from build123d import *

# Parameters (mm, degrees)
SKETCH_1_R          = 15
EXTRUDE_1_DEPTH     = 5.65
SKETCH_2_R          = 10
EXTRUDE_2_DEPTH     = 46.4
SKETCH_3_R          = 1.25
CUT_EXTRUDE_1_DEPTH = 10
SKETCH_4_OUTSIDE_W  = 45.43
SKETCH_4_OUTSIDE_H  = 45.43
SKETCH_4_OUTSIDE_R  = 7.5
CUT_EXTRUDE_2_DEPTH = 7
SKETCH_5_OUTSIDE_W  = 45.43
SKETCH_5_OUTSIDE_H  = 45.43
SKETCH_5_OUTSIDE_R  = 8.5
CUT_EXTRUDE_3_DEPTH = 1
SKETCH_6_R          = 1.4
CUT_EXTRUDE_4_DEPTH = 8
CUT_EXTRUDE_5_DEPTH = 3


with BuildPart() as part:
    # 草图1 → 凸台-拉伸1 (new body)
    with BuildSketch(Plane.XY):
        Circle(SKETCH_1_R)
    extrude(amount=EXTRUDE_1_DEPTH)

    # 草图2 → 凸台-拉伸2 (add)
    with BuildSketch(Plane.XY.offset(5.65)):
        Circle(SKETCH_2_R)
    extrude(amount=EXTRUDE_2_DEPTH)

    # 草图3 → 切除-拉伸1 (cut)
    with BuildSketch(Plane(origin=(0, 0, 0), x_dir=(-1, 0, 0), z_dir=(0, 0, -1))):
        with Locations((0, 7)):
            Circle(SKETCH_3_R)
        with Locations((7, 0)):
            Circle(SKETCH_3_R)
        with Locations((0, -7)):
            Circle(SKETCH_3_R)
        with Locations((-7, 0)):
            Circle(SKETCH_3_R)
    extrude(amount=-CUT_EXTRUDE_1_DEPTH, mode=Mode.SUBTRACT)

    # 草图4 outside → 切除-拉伸2 (cut)
    with BuildSketch(Plane.XY.offset(52.05)):
        Rectangle(SKETCH_4_OUTSIDE_W, SKETCH_4_OUTSIDE_H)
        Circle(SKETCH_4_OUTSIDE_R, mode=Mode.SUBTRACT)
    extrude(amount=-CUT_EXTRUDE_2_DEPTH, mode=Mode.SUBTRACT)

    # 草图5 outside → 切除-拉伸3 (cut)
    with BuildSketch(Plane.XY.offset(45.05)):
        Rectangle(SKETCH_5_OUTSIDE_W, SKETCH_5_OUTSIDE_H)
        Circle(SKETCH_5_OUTSIDE_R, mode=Mode.SUBTRACT)
    extrude(amount=-CUT_EXTRUDE_3_DEPTH, mode=Mode.SUBTRACT)

    # 草图6 → 切除-拉伸4 (cut)
    with BuildSketch(Plane(origin=(0, 10, 0), x_dir=(1, 0, 0), z_dir=(0, 1, 0))):
        with Locations(Location((0, -39.65, 0), (0, 0, 270))):
            Circle(SKETCH_6_R)
    cut_extrude_4 = extrude(amount=-CUT_EXTRUDE_4_DEPTH, mode=Mode.SUBTRACT)

    # 镜向1: 切除-拉伸4 across plane
    add(cut_extrude_4.mirror(Plane.ZX), mode=Mode.SUBTRACT)

    # 草图7 → 切除-拉伸5 (cut)
    with BuildSketch(Plane(origin=(10, 0, 0), x_dir=(0, 0, -1), z_dir=(1, 0, 0))):
        with BuildLine():
            Line((-32.15, 2.6), (-15.65, 2.6))
            ThreePointArc((-15.65, 2.6), (-13.05, 0), (-15.65, -2.6))
            Line((-15.65, -2.6), (-32.15, -2.6))
            ThreePointArc((-32.15, -2.6), (-34.75, 0), (-32.15, 2.6))
        make_face()
    extrude(amount=-CUT_EXTRUDE_5_DEPTH, mode=Mode.SUBTRACT)


solid = part.part
Could you check a few things on this model? Use its own coordinates, in mm. A direction names the side the tool comes from. Round coordinates to 2 decimals unless told otherwise and drop trailing zeros. Order: outer loops, then holes, each group sorted by start corner. A loop starts at its lowest first (then second) coordinate and runs counter-clockwise, first axis right, second up.
(1) Please list where these lines run through material, in increasing order: line 1 along Z through (x, y) = (0, -7.75); line 2 along X through (y, z) = (-5.25, 39.65); line 3 along Z through (x, y) = (12, -0.5).
Response values:
line 1: z = 10 to 38.25, 41.05 to 45.05
line 2: x = -8.51 to -1.4, 1.4 to 8.51
line 3: z = 0 to 5.65
(2) Imagine slicing it at D-D (z = 25.5). Write out the boundary of the cut face in (x, y), plus the area to 3 significant figures.
Response values:
outline: (7, -2.6) - (7, 2.6) - (9.66, 2.6) arc R10 ccw (long way) to (9.66, -2.6) - close
area: 299 mm2
(3) Imagine slicing it at B-B (z = 36.5). Write out the boundary of the cut face in (x, y).
Response values:
outline: circle Ø20 at (0, 0)
(4) Which directions (+Z, -Z, +X, -X, +Y, -Y) give clear straight access to the entire face, cutting with the end or side of a thin tool? Please do faces 1 (the cylindrical face through (-14.985, 0.66, 2.785)), 2 (the cylindrical face through (0.27, 5.78, 4.93)), 3 (the flat face through (0, 0, 0)), 4 (the cylindrical face through (8.52, -0.06, 34.75)), 5 (the cylindrical face through (-2.17, -9.76, 24.58)).
Response values:
face 1: +Z, -Z
face 2: -Z
face 3: -Z, +X, -X, +Y, -Y
face 4: +X
face 5: +Z
(5) I'm going to push flat-ended pins straight in: pin 1 (2 mm diameter, centred on x = -0.5, z = 40, fed in from -Y); pin 2 (10 mm diameter, centred on x = 5.5, y = 6, fed in from -Z); pin 3 (3.5 mm diameter, centred on x = 0, z = 39.65, fed in from +Y); pin 4 (1.7 mm diameter, centred on x = 0, z = 39.65, fed in from +Y). Where does each tip first touch, or does it pass through?
Response values:
pin 1: stops at y = -9.99
pin 2: stops at z = 0
pin 3: stops at y = 10
pin 4: stops at y = 2
(6) If we mould it in two halves opening along Y, with no side actions, what happens to faces 6 (the flat face through (8, 2.6, 24)), 7 (the cylindrical face through (0.421, -6.056, 40.985)), 8 (the cylindrical face through (-7.493, 0.33, 48.599))? For each: released by +Y, released by -Y, zero draft, split by the parting line, or undercut.
Response values:
face 6: undercut
face 7: zero draft
face 8: split by the parting line
(7) Imagine slicing it at C-C (x = -3.25). Write out the boundary of the cut face in (y, z).
Response values:
outline: (-14.64, 0) - (14.64, 0) - (14.64, 5.65) - (9.46, 5.65) - (9.46, 44.05) - (7.85, 44.05) - (7.85, 45.05) - (6.76, 45.05) - (6.76, 52.05) - (-6.76, 52.05) - (-6.76, 45.05) - (-7.85, 45.05) - (-7.85, 44.05) - (-9.46, 44.05) - (-9.46, 5.65) - (-14.64, 5.65) - close
